The model under review builds one solid part; all positions refer to its coordinate system, in mm. A direction names the side the tool comes from. Coordinates: 2 decimals unless noted, no trailing zeros. Write each loop counter-clockwise with the first axis right and the second up, starting at its lowest first coordinate (ties: lowest second). Pieces come first, ordered by that corner, then holes.
1) Add section B-B, the plane z = 11.04. State the section outline as (x, y) points.
2) For line 1 (Z direction, x = 5, y = 10.2); line 2 (X direction, y = 9.9, z = 11.04); line 3 (Y direction, x = 1, z = 16.5), list the stretches that pass through material, from the lowest coordinate up.
3) Add section A-A, the plane x = -3. State the section outline as (y, z) points.
4) Machinability: for faces 1 (the cylindrical face through (-1.57, 0.25, 2.27)), 2 (the flat face through (1, 9.104, 18)), which of the approach directions +Z, -Z, +X, -X, +Y, -Y give a long, thin tool a straight path to every point of the face, cutting with its end or side? Answer none if there is none.
5) For P1, Ø6, axis at x = -3, z = 12.5, coming from the -Y side; P2, Ø6.5, axis at x = 2, y = 1, coming from the +Z side, all flat-tipped, find the tip position at first contact; note any pin that passes through.
6) Mouldability with a two-part tool opening along Z and no side actions: class faces 3 (the flat face through (-5.5, 10, 9)), 4 (the flat face through (1, 10, 31.6)), 5 (the cylindrical face through (4.93, 9.84, 24.54)), 6 (the cylindrical face through (-3.07, 9.84, 18.54)) as released by +Z, released by -Z, zero draft, split by the parting line, or undercut.
7) Add section C-C, the plane x = 2.25. State the section outline as (y, z) points, then the cut area to 3 significant figures.
from build123d import *

# Parameters (mm, degrees)
SKETCH2_W           = 13
SKETCH2_H           = 12.3
SKETCH2_R           = 1.5
BOSS_EXTRUDE1_DEPTH = 4.6
SKETCH3_W           = 13
SKETCH3_H           = 27
SKETCH3_R           = 1.5
BOSS_EXTRUDE2_DEPTH = 10.603673126
SKETCH4_W           = 13
SKETCH4_H           = 12.3
CUT_EXTRUDE1_DEPTH  = 27
SKETCH5_W           = 13
SKETCH5_H           = 3
BOSS_EXTRUDE3_DEPTH = 4.6
SKETCH7_W           = 13
SKETCH7_H           = 27
CUT_EXTRUDE2_DEPTH  = 1.5


with BuildPart() as part:
    # Sketch2 → Boss-Extrude1 (new body)
    with BuildSketch(Plane.XY):
        with Locations((1, 1.453673126)):
            Rectangle(SKETCH2_W, SKETCH2_H)
        with Locations((-3, 5.803673126)):
            Circle(SKETCH2_R, mode=Mode.SUBTRACT)
        with Locations((-3, -0.196326874)):
            Circle(SKETCH2_R, mode=Mode.SUBTRACT)
        with Locations(Location((5, -0.196326874, 0), (0, 0, 180))):
            Circle(SKETCH2_R, mode=Mode.SUBTRACT)
        with Locations(Location((5, 5.803673126, 0), (0, 0, 180))):
            Circle(SKETCH2_R, mode=Mode.SUBTRACT)
    extrude(amount=BOSS_EXTRUDE1_DEPTH)

    # Sketch3 → Boss-Extrude2 (add)
    with BuildSketch(Plane(origin=(0, 0, 0), x_dir=(1, 0, 0), z_dir=(0, 1, 0))):
        with Locations((1, -18.1)):
            Rectangle(SKETCH3_W, SKETCH3_H)
        with Locations(Location((-3, -17.04, 0), (0, 0, 90))):
            Circle(SKETCH3_R, mode=Mode.SUBTRACT)
        with Locations(Location((-3, -23.04, 0), (0, 0, 90))):
            Circle(SKETCH3_R, mode=Mode.SUBTRACT)
        with Locations(Location((5, -23.04, 0), (0, 0, 90))):
            Circle(SKETCH3_R, mode=Mode.SUBTRACT)
        with Locations(Location((5, -17.04, 0), (0, 0, 90))):
            Circle(SKETCH3_R, mode=Mode.SUBTRACT)
        with Locations(Location((-3, -11.04, 0), (0, 0, 90))):
            Circle(SKETCH3_R, mode=Mode.SUBTRACT)
        with Locations(Location((5, -11.04, 0), (0, 0, 90))):
            Circle(SKETCH3_R, mode=Mode.SUBTRACT)
    extrude(amount=BOSS_EXTRUDE2_DEPTH)

    # Sketch4 → Cut-Extrude1 (cut)
    with BuildSketch(Plane.XY.offset(31.6)):
        with Locations((1, 1.453673126)):
            Rectangle(SKETCH4_W, SKETCH4_H)
    extrude(amount=-CUT_EXTRUDE1_DEPTH, mode=Mode.SUBTRACT)


with BuildPart() as cut_extrude1_piece_1:
    # of the separate pieces the step leaves, piece 1, a body of its own (cut_extrude1_pieces)
    add(part.part.solids().sort_by_distance((7.5, 10.603673126, 4.6))[0])



with BuildPart() as cut_extrude1_piece_2:
    # of the separate pieces the step leaves, piece 2, a body of its own (cut_extrude1_pieces)
    add(part.part.solids().sort_by_distance((-5.5, 7.603673126, 0))[0])


with BuildPart() as cut_extrude1_piece_1_1:
    add(cut_extrude1_piece_1.part)

    add(cut_extrude1_piece_2.part)  # Boss-Extrude3 merges Cut-Extrude1 piece 2
    # Sketch5 → Boss-Extrude3 (add)
    with BuildSketch(Plane(origin=(0, 0, 4.6), x_dir=(-1, 0, 0), z_dir=(0, 0, -1))):
        with Locations((-1, 9.103673126)):
            Rectangle(SKETCH5_W, SKETCH5_H)
    extrude(amount=BOSS_EXTRUDE3_DEPTH)

    # Sketch7 → Cut-Extrude2 (cut)
    with BuildSketch(Plane.XZ.offset(-7.603673126)):
        with Locations((1, 18.1)):
            Rectangle(SKETCH7_W, SKETCH7_H)
    extrude(amount=-CUT_EXTRUDE2_DEPTH, mode=Mode.SUBTRACT)


solid = cut_extrude1_piece_1_1.part
Geometry results:
1. outline: (-5.5, 9.1) - (-4.5, 9.1) - (-4.5, 10.6) - (-5.5, 10.6) - close; (-1.5, 9.1) - (3.5, 9.1) - (3.5, 10.6) - (-1.5, 10.6) - close; (6.5, 9.1) - (7.5, 9.1) - (7.5, 10.6) - (6.5, 10.6) - close
2. line 1: z = 0 to 9.54, 12.54 to 15.54, 18.54 to 21.54, 24.54 to 31.6
2. line 2: x = -5.5 to -4.5, -1.5 to 3.5, 6.5 to 7.5
2. line 3: y = 9.1 to 10.6
3. outline: (-4.7, 0) - (-1.7, 0) - (-1.7, 4.6) - (-4.7, 4.6) - close; (1.3, 0) - (4.3, 0) - (4.3, 4.6) - (1.3, 4.6) - close; (7.3, 0) - (10.6, 0) - (10.6, 9.54) - (9.1, 9.54) - (9.1, 4.6) - (7.3, 4.6) - close; (9.1, 12.54) - (10.6, 12.54) - (10.6, 15.54) - (9.1, 15.54) - close; (9.1, 18.54) - (10.6, 18.54) - (10.6, 21.54) - (9.1, 21.54) - close; (9.1, 24.54) - (10.6, 24.54) - (10.6, 31.6) - (9.1, 31.6) - close
4. face 1: +Z, -Z
4. face 2: +Z, +X, -X, -Y
5. P1: stops at y = 9.1
5. P2: stops at z = 4.6
6. face 3: zero draft
6. face 4: released by +Z
6. face 5: undercut
6. face 6: undercut
7. outline: (-4.7, 0) - (10.6, 0) - (10.6, 31.6) - (9.1, 31.6) - (9.1, 4.6) - (-4.7, 4.6) - close
7. area: 111 mm2
